Could you check a few things on this drawing? It's one solid part, dimensions in mm from its lowest x, y, z. A direction names the side the tool comes from. Give positions to 0.01 mm unless a question says otherwise; leave off trailing zeros. Order: outer loops, then holes, each group sorted by start corner. A loop starts at its lowest first (then second) coordinate and runs counter-clockwise, first axis right, second up. Notation, with made-up numbers: (44.5, 31.5) -> (65.5, 31.5) arc R11 cw to (65.5, 41.5) -> close; hole circle Ø2 at (-35.5, 19). An arc over 180 degrees is marked (long way). Answer as a JSON object with one key per item and string values.
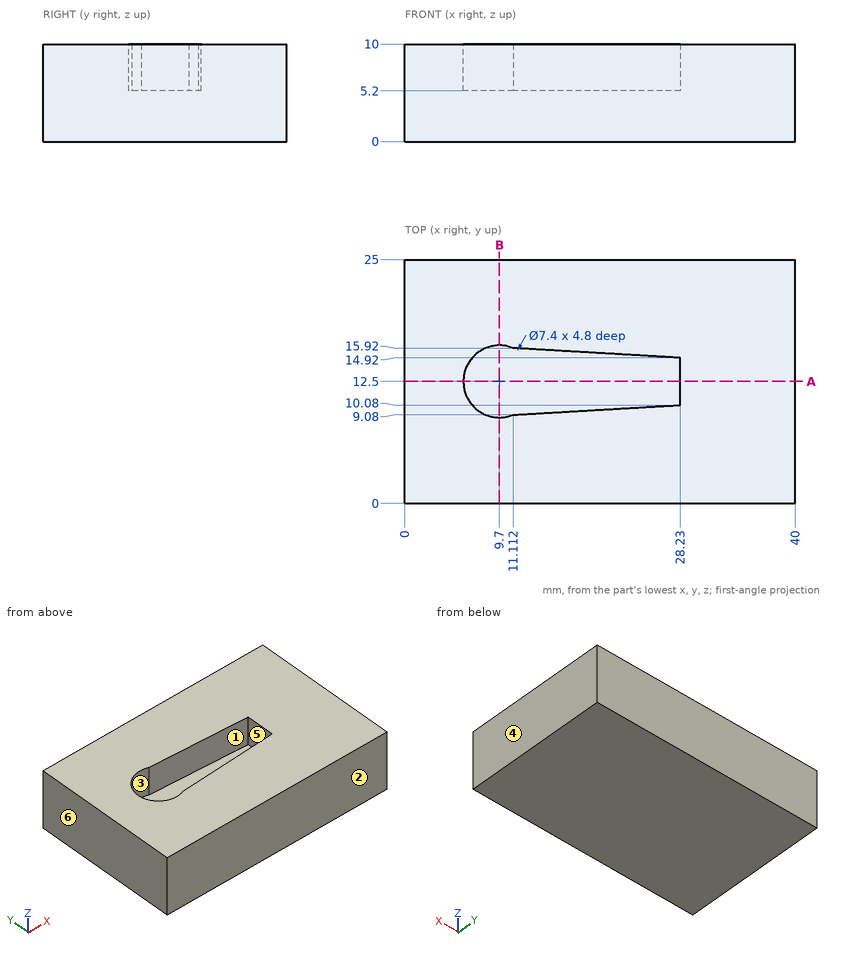
1. Please list where these lines run through material, in increasing order: L1, parallel to X at y = 12.5, z = 6.2; L2, parallel to Y at x = 9.7, z = 6.6; L3, parallel to Z at x = 8, y = 15.75.
Worked answers:
{"L1": "0 to 6, 28.23 to 40", "L2": "0 to 8.8, 16.2 to 25", "L3": "0 to 5.2"}
2. Will this pin go through, and if not, where does the flat tip stop? pin 1 Ø3.5 at (x, y) = (20, 13) entering from +Z.
Worked answers:
{"pin 1": "z = 5.2"}
3. If we section it at A-A on y = 12.5: Please give me the cut outline in (x, z).
Worked answers:
{"outline": "(0, 0) -> (40, 0) -> (40, 10) -> (28.23, 10) -> (28.23, 5.2) -> (6, 5.2) -> (6, 10) -> (0, 10) -> close"}
4. If we mould it in two halves opening along X, with no side actions, what happens to the marked faces 1, 2, 3 and 4? For each: +X half, -X half, draft (parallel to the pull), parting line (faces both ways), or undercut.
Worked answers:
{"face 1": "undercut", "face 2": "draft", "face 3": "undercut", "face 4": "+X half"}
5. If we section it at B-B on x = 9.7: Please give me the cut outline in (y, z), then the cut area to 3 significant figures.
Worked answers:
{"outline": "(0, 0) -> (25, 0) -> (25, 10) -> (16.2, 10) -> (16.2, 5.2) -> (8.8, 5.2) -> (8.8, 10) -> (0, 10) -> close", "area": "214 mm²"}
6. For the marked faces 5 and 6, which set-ups out of +Z, -Z, +X, -X, +Y, -Y let a thin tool reach every point of the face, with its end or its side?
Worked answers:
{"face 5": "+Z", "face 6": "+Z, -Z, -X, +Y, -Y"}
